from build123d import *

# Parameters (mm, degrees)
F0_R        = 10.011227
F0_R_2      = 7.627377
F2_DEPTH    = 25
F2_FACE_R   = 10.011227
F2_FACE_R_2 = 7.627377
F5_DEPTH    = 6


with BuildPart() as f2:
    # F0 (on Front) → F2 (new body, symmetric)
    with BuildSketch(Plane.XZ):
        Circle(F0_R)
        Circle(F0_R_2, mode=Mode.SUBTRACT)
    extrude(amount=F2_DEPTH, both=True)

    # F3 (on Right) → F4 (revolve)
    with BuildSketch(Plane.YZ):
        Polygon((-23.677679, -10.02051), (-23.677679, -7.532166), (-38.399562, 0), (-43.263118, 0), align=None)
    revolve(axis=Axis((0, -31.038621, 0), (0, 1, 0)))

    # F2_face (on face) → F5 (join)
    with BuildSketch(Plane(origin=(0, 25, 0), x_dir=(1, 0, 0), z_dir=(0, 1, 0))):
        Circle(F2_FACE_R)
        Circle(F2_FACE_R_2, mode=Mode.SUBTRACT)
    extrude(amount=F5_DEPTH)


solid = f2.part
Here's how the part is built. I have some questions about the finished solid (model axes, mm). Coordinates: 2 decimals unless noted, no trailing zeros. Order: outer loops, then holes, each group sorted by start corner. A loop starts at its lowest first (then second) coordinate and runs counter-clockwise, first axis right, second up. Notation, with made-up numbers: (53, 23.5) -> (73, 23.5) arc R10 ccw to (73, 36.5) -> close; hole circle Ø10 at (-22, 55.25). An arc over 180 degrees is marked (long way). Answer in a Markdown table with one row per item.
(1) Thinking about a two-plate mould opening in Z: for faces 1 (the face through (-1.653, 3.278, 7.446)), 2 (the face through (-7, 31, 4)), 3 (the face through (9.55, -24.36, 3.01)), which applies, +Z half, -Z half, draft (parallel to the pull), parting line (faces both ways), or undercut?
Answer key:
| item | result |
|---|---|
| face 1 | undercut |
| face 2 | draft |
| face 3 | parting line |
(2) Will these pins go through, and if not, where does the flat tip stop? pin 1 Ø1.5 at (x, z) = (-5, 0) entering from -Y; pin 2 Ø12 at (y, z) = (18, -8) entering from +X; pin 3 Ø4 at (x, z) = (-6, 6.5) entering from -Y.
Answer key:
| item | result |
|---|---|
| pin 1 | y = -34.96 |
| pin 2 | x = 9.81 |
| pin 3 | y = -29.88 |
(3) I want a section at B-B on y = -30. List the corners of the cut face in (x, z) for me.
Answer key:
| item | result |
|---|---|
| outline | circle Ø13.57 at (0, 0); hole circle Ø8.59 at (0, 0) |
(4) Please list where these lines run through material, in increasing order: probe 1 along X at (y, z) = (0.5, 0); probe 2 along X at (y, z) = (-6.5, 1.25).
Answer key:
| item | result |
|---|---|
| probe 1 | -10.01 to -7.63, 7.63 to 10.01 |
| probe 2 | -9.93 to -7.52, 7.52 to 9.93 |
(5) I want a section at A-A on y = -20.5. List the corners of the cut face in (x, z) for me, then the cut area to 3 significant figures.
Answer key:
| item | result |
|---|---|
| outline | circle Ø20.02 at (0, 0); hole circle Ø15.25 at (0, 0) |
| area | 132 mm^2 |
